Geometry check sheet. Reference: the model listing, model coordinates, mm. Face numbers are marked on the shaded views. Round coordinates to 2 decimals unless told otherwise and drop trailing zeros. Order: outer loops, then holes, each group sorted by start corner. A loop starts at its lowest first (then second) coordinate and runs counter-clockwise, first axis right, second up. Notation, with made-up numbers: (77, -34.75) - (90, -34.75) arc R10 ccw to (90, -20.75) - close; hole circle Ø9 at (-36.5, 42). An arc over 180 degrees is marked (long way). One line per question, with ' | ' between items. Start each with the question number.
Q1. Sectioned sample at D-D, the plane z = 0.5. Enter the section's corners in (x, y).
Q2. Material ranges on line 1 along X through (y, z) = (68.64, 0.65); line 2 along Y through (x, z) = (-40.5, 1.15); line 3 along Y through (x, z) = (-32, 0.9), recorded low to high.
Q3. Sectioned sample at A-A, the plane x = -4. Give the number of separate pieces and of enclosed holes in the cut face, then the cut area to 3 significant figures.
Q4. Gauge pin test, flat ends, axial feed: P1, Ø3, axis at x = -4, y = 68.64, coming from the +Z side; P2, Ø0.5, axis at x = -25, z = 0.5, coming from the +Y side; P3, Ø0.5, axis at x = -15.5, z = 1.5, coming from the +Y side; P4, Ø12, axis at x = -15, y = 30.5, coming from the -Z side. Record the tip position at first contact, or that the pin passes through.
Q5. Sectioned sample at B-B, the plane y = 68.64. Enter the section's corners in (x, z), then the cut area to 3 significant figures.
Q6. Mould release check, pull along X, two halves, no side actions. Record for the marked faces 1 and 2: +X half, -X half, draft (parallel to the pull), parting line (faces both ways), or undercut.
Q7. Sectioned sample at C-C, the plane y = 49. Enter the section's corners in (x, z), then the cut area to 3 significant figures.
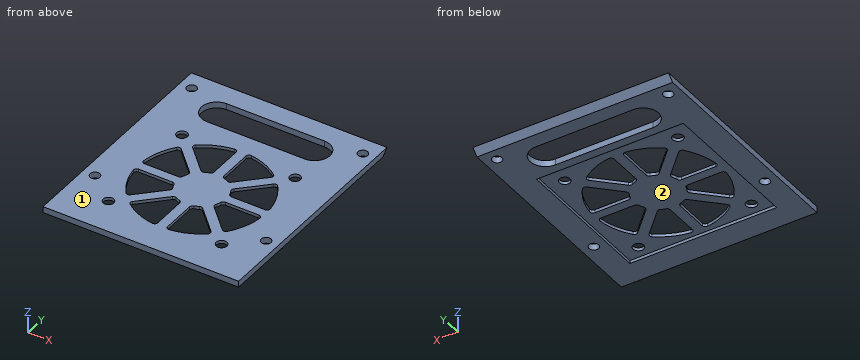
```python
from build123d import *

# Parameters (mm, degrees)
SZKIC1_W                    = 64
SZKIC1_H                    = 2
SZKIC1_H_2                  = 72.64
DODANIE_WYCI_GNI_CIE1_DEPTH = 2
SFAZOWANIE1_SIZE            = 2
SZKIC2_R                    = 1.6
WYTNIJ_WYCI_GNI_CIE1_DEPTH  = 2
WYTNIJ_WYCI_GNI_CIE2_DEPTH  = 10
ZAOKR_GLENIE1_R             = 1
SZKIC4_R                    = 1.75
WYTNIJ_WYCI_GNI_CIE3_DEPTH  = 10
WYTNIJ_WYCI_GNI_CIE4_DEPTH  = 10
SZKIC6_W                    = 48
SZKIC6_H                    = 47
WYTNIJ_WYCI_GNI_CIE5_DEPTH  = 1


with BuildPart() as part:
    # Szkic1 → Dodanie-wyciągnięcie1 (new body)
    with BuildSketch(Plane.XY):
        with Locations((-32, 73.64)):
            Rectangle(SZKIC1_W, SZKIC1_H)
        with Locations((-32, 36.32)):
            Rectangle(SZKIC1_W, SZKIC1_H_2)
    extrude(amount=DODANIE_WYCI_GNI_CIE1_DEPTH)

    # Sfazowanie1
    sfazowanie1_edges = [part.edges().sort_by_distance(p)[0] for p in [
        (-32, 74.64, 0),
    ]]
    chamfer(sfazowanie1_edges, length=SFAZOWANIE1_SIZE - 0.0001)  # a hair under: the kernel refuses the full size

    # Szkic2 → Wytnij-wyciągnięcie1 (cut)
    with BuildSketch(Plane.XY.offset(2)):
        with Locations((-60, 20)):
            Circle(SZKIC2_R)
        with Locations((-4, 20)):
            Circle(SZKIC2_R)
        with Locations((-4, 68.64)):
            Circle(SZKIC2_R)
        with Locations((-60, 68.64)):
            Circle(SZKIC2_R)
    extrude(amount=-WYTNIJ_WYCI_GNI_CIE1_DEPTH, mode=Mode.SUBTRACT)

    # Szkic3 → Wytnij-wyciągnięcie2 (cut)
    with BuildSketch(Plane(origin=(0, 0, 0), x_dir=(-1, 0, 0), z_dir=(0, 0, -1))):
        with BuildLine():
            Line((11.056403618, 32), (24.016552746, 32))
            ThreePointArc((24.016552746, 32), (24.466137465, 33.518882587), (25.206174928, 34.919409376))
            Line((25.206174928, 34.919409376), (16.034132153, 44.091452151))
            ThreePointArc((16.034132153, 44.091452151), (12.573950156, 38.445591693), (11.056403618, 32))
        make_face()
        with BuildLine():
            ThreePointArc((25.206174928, 26.080590624), (24.466137465, 27.481117413), (24.016552746, 29))
            Line((24.016552746, 29), (11.056403618, 29))
            ThreePointArc((11.056403618, 29), (12.573950156, 22.554408307), (16.034132153, 16.908547849))
            Line((16.034132153, 16.908547849), (25.206174928, 26.080590624))
        make_face()
        with BuildLine():
            ThreePointArc((27.455260193, 37.168494641), (28.795563732, 37.883705523), (30.246904647, 38.332648426))
            Line((30.246904647, 38.332648426), (30.246904647, 51.308665948))
            ThreePointArc((30.246904647, 51.308665948), (23.86987617, 49.77624133), (18.283217418, 46.340537416))
            Line((18.283217418, 46.340537416), (27.455260193, 37.168494641))
        make_face()
        with BuildLine():
            ThreePointArc((33.50243449, 38.332648426), (34.953775405, 37.883705523), (36.294078944, 37.168494641))
            Line((36.294078944, 37.168494641), (45.466121719, 46.340537416))
            ThreePointArc((45.466121719, 46.340537416), (39.879462967, 49.77624133), (33.50243449, 51.308665948))
            Line((33.50243449, 51.308665948), (33.50243449, 38.332648426))
        make_face()
        with BuildLine():
            ThreePointArc((38.543164209, 34.919409376), (39.283201672, 33.518882587), (39.732786391, 32))
            Line((39.732786391, 32), (52.692935519, 32))
            ThreePointArc((52.692935519, 32), (51.175388981, 38.445591693), (47.715206984, 44.091452151))
            Line((47.715206984, 44.091452151), (38.543164209, 34.919409376))
        make_face()
        with BuildLine():
            Line((52.692935519, 29), (39.732786391, 29))
            ThreePointArc((39.732786391, 29), (39.283201672, 27.481117413), (38.543164209, 26.080590624))
            Line((38.543164209, 26.080590624), (47.715206984, 16.908547849))
            ThreePointArc((47.715206984, 16.908547849), (51.175388981, 22.554408307), (52.692935519, 29))
        make_face()
        with BuildLine():
            Line((45.466121719, 14.659462584), (36.294078944, 23.831505359))
            ThreePointArc((36.294078944, 23.831505359), (34.953775405, 23.116294477), (33.50243449, 22.667351574))
            Line((33.50243449, 22.667351574), (33.50243449, 9.691334052))
            ThreePointArc((33.50243449, 9.691334052), (39.879462967, 11.22375867), (45.466121719, 14.659462584))
        make_face()
        with BuildLine():
            Line((30.246904647, 9.691334052), (30.246904647, 22.667351574))
            ThreePointArc((30.246904647, 22.667351574), (28.795563732, 23.116294477), (27.455260193, 23.831505359))
            Line((27.455260193, 23.831505359), (18.283217418, 14.659462584))
            ThreePointArc((18.283217418, 14.659462584), (23.86987617, 11.22375867), (30.246904647, 9.691334052))
        make_face()
    extrude(amount=-WYTNIJ_WYCI_GNI_CIE2_DEPTH, mode=Mode.SUBTRACT)

    # Zaokrąglenie1
    zaokr_glenie1_edges = [part.edges().sort_by_distance(p)[0] for p in [
        (-36.294078944, 37.168494641, 1),
        (-33.50243449, 38.332648426, 1),
        (-33.50243449, 51.308665948, 1),
        (-45.466121719, 46.340537416, 1),
        (-33.50243449, 22.667351574, 1),
        (-36.294078944, 23.831505359, 1),
        (-45.466121719, 14.659462584, 1),
        (-33.50243449, 9.691334052, 1),
        (-38.543164209, 26.080590624, 1),
        (-39.732786391, 29, 1),
        (-52.692935519, 29, 1),
        (-47.715206984, 16.908547849, 1),
        (-27.455260193, 23.831505359, 1),
        (-30.246904647, 22.667351574, 1),
        (-30.246904647, 9.691334052, 1),
        (-18.283217418, 14.659462584, 1),
        (-25.206174928, 34.919409376, 1),
        (-24.016552746, 32, 1),
        (-11.056403618, 32, 1),
        (-16.034132153, 44.091452151, 1),
        (-24.016552746, 29, 1),
        (-25.206174928, 26.080590624, 1),
        (-16.034132153, 16.908547849, 1),
        (-11.056403618, 29, 1),
        (-30.246904647, 38.332648426, 1),
        (-27.455260193, 37.168494641, 1),
        (-18.283217418, 46.340537416, 1),
        (-30.246904647, 51.308665948, 1),
        (-39.732786391, 32, 1),
        (-38.543164209, 34.919409376, 1),
        (-47.715206984, 44.091452151, 1),
        (-52.692935519, 32, 1),
    ]]
    fillet(zaokr_glenie1_edges, radius=ZAOKR_GLENIE1_R)

    # Szkic4 → Wytnij-wyciągnięcie3 (cut)
    with BuildSketch(Plane(origin=(0, 0, 0), x_dir=(-1, 0, 0), z_dir=(0, 0, -1))):
        with Locations((13.374669569, 49)):
            Circle(SZKIC4_R)
        with Locations((50.374669569, 49)):
            Circle(SZKIC4_R)
        with Locations((50.374669569, 12)):
            Circle(SZKIC4_R)
        with Locations((13.374669569, 12)):
            Circle(SZKIC4_R)
    extrude(amount=-WYTNIJ_WYCI_GNI_CIE3_DEPTH, mode=Mode.SUBTRACT)

    # Szkic5 → Wytnij-wyciągnięcie4 (cut)
    with BuildSketch(Plane(origin=(0, 0, 0), x_dir=(-1, 0, 0), z_dir=(0, 0, -1))):
        with BuildLine():
            Line((16.000918864, 67.82), (48, 67.82))
            ThreePointArc((48, 67.82), (53, 62.82), (48, 57.82))
            Line((48, 57.82), (16.000918864, 57.82))
            ThreePointArc((16.000918864, 57.82), (11.000918864, 62.82), (16.000918864, 67.82))
        make_face()
    extrude(amount=-WYTNIJ_WYCI_GNI_CIE4_DEPTH, mode=Mode.SUBTRACT)

    # Szkic6 → Wytnij-wyciągnięcie5 (cut)
    with BuildSketch(Plane(origin=(0, 0, 0), x_dir=(-1, 0, 0), z_dir=(0, 0, -1))):
        with Locations((32, 31.5)):
            Rectangle(SZKIC6_W, SZKIC6_H)
    extrude(amount=-WYTNIJ_WYCI_GNI_CIE5_DEPTH, mode=Mode.SUBTRACT)


solid = part.part
```
Determined:
1) outline: (-64, 0) - (0, 0) - (0, 73.14) - (-64, 73.14) - close; hole circle Ø3.2 at (-60, 20); hole circle Ø3.2 at (-60, 68.64); hole (-56, 8) - (-8, 8) - (-8, 55) - (-56, 55) - close; hole (-48, 57.82) - (-16, 57.82) arc R5 ccw to (-16, 67.82) - (-48, 67.82) arc R5 ccw to start; hole circle Ø3.2 at (-4, 20); hole circle Ø3.2 at (-4, 68.64)
2) line 1: x = -64 to -61.6, -58.4 to -5.6, -2.4 to 0 | line 2: y = 0 to 11.49, 19.63 to 24.12, 29 to 32, 36.88 to 41.37, 49.51 to 57.82, 67.82 to 73.79 | line 3: y = 0 to 8, 55 to 57.82, 67.82 to 73.54
3) separate pieces: 3 | enclosed holes: 0 | area: 134 mm2
4) P1: passes through | P2: stops at y = 73.39 | P3: stops at y = 74.39 | P4: stops at z = 1
5) outline: (-64, 0) - (-61.6, 0) - (-61.6, 2) - (-64, 2) - close; (-58.4, 0) - (-5.6, 0) - (-5.6, 2) - (-58.4, 2) - close; (-2.4, 0) - (0, 0) - (0, 2) - (-2.4, 2) - close | area: 115 mm2
6) face 1: draft | face 2: undercut
7) outline: (-64, 0) - (-56, 0) - (-56, 1) - (-52.12, 1) - (-52.12, 2) - (-64, 2) - close; (-48.62, 1) - (-41.54, 1) - (-41.54, 2) - (-48.62, 2) - close; (-33.5, 1) - (-30.25, 1) - (-30.25, 2) - (-33.5, 2) - close; (-22.21, 1) - (-15.12, 1) - (-15.12, 2) - (-22.21, 2) - close; (-11.62, 1) - (-8, 1) - (-8, 0) - (0, 0) - (0, 2) - (-11.62, 2) - close | area: 56.9 mm2
